Work out the finished part from the listing and answer in its coordinate system (mm). Give positions to 0.01 mm unless a question says otherwise; leave off trailing zeros. Write each loop counter-clockwise with the first axis right and the second up, starting at its lowest first coordinate (ties: lowest second). Pieces come first, ordered by that corner, then holes. Notation, with made-up numbers: (38, 85) -> (46, 85) arc R21 ccw to (46, 118) -> close; hole circle Ø2 at (-8.75, 43.25). An arc over 180 degrees is marked (long way). Use a Markdown table: item, result. Add a question column.
Q1. For a pull along Y with two mould halves and no side action, classify faces 1 (the face through (-11.012, -49.592, 3.131)), 2 (the face through (-1, 1, 0)), 3 (the face through (36, -8.466, 3)), 4 (the face through (12, -29.209, 3)) as pulls with the +Y half, pulls with the -Y half, needs draft (parallel to the pull), parting line crosses it, or undercut.
Q2. Section A-A, the plane x = 0 is taken. Give the vertices of the cut face in (y, z), plus the area to 3 significant figures.
Q3. Section C-C, the plane y = 17 is taken. Give the vertices of the cut face in (x, z), plus the area to 3 significant figures.
Q4. Consider line 1 (Y direction, x = 15.5, z = 1); line 2 (Y direction, x = 29.5, z = 3.25); line 3 (Y direction, x = 38, z = 3.75). Determine where each line is inside the solid, lowest interval first.
Q5. Each of these flat-tipped pins is pushed along its axis until it touches: pin 1 Ø3 at (x, z) = (35, 3.5) entering from +Y; pin 2 Ø3 at (y, z) = (19.5, 4) entering from -X; pin 3 Ø2 at (x, z) = (-18.5, 4.5) entering from +Y. Where does it stop, or does it pass through?
Q6. Section D-D, the plane x = 11 is taken. Give the vertices of the cut face in (y, z), plus the area to 3 significant figures.
Q7. Section B-B, the plane z = 4.25 is taken. State how many separate pieces and enclosed holes the cut face has, plus the area to 3 significant figures.
from build123d import *

# Parameters (mm, degrees)
SKETCH1_R           = 50.8
BOSS_EXTRUDE1_DEPTH = 6.35
SKETCH2_W           = 19.230854478
SKETCH2_H           = 28.543909792
SKETCH2_W_2         = 18.081841161
SKETCH2_H_2         = 27.999640326
SKETCH2_W_3         = 10.22017109
SKETCH2_H_3         = 7.559298144
SKETCH2_W_4         = 8.829260232
SKETCH2_H_4         = 7.256926218
SKETCH2_W_5         = 9.97827355
SKETCH2_H_5         = 8.164041996
SKETCH2_W_6         = 10.703966172
SKETCH2_H_6         = 6.531233596
SKETCH2_W_7         = 12.336774571
SKETCH2_H_7         = 9.04092058
SKETCH2_W_8         = 11.127286868
SKETCH2_H_8         = 7.7407213
CUT_EXTRUDE1_DEPTH  = 73.122135992


with BuildPart() as part:
    # Sketch1 → Boss-Extrude1 (new body)
    with BuildSketch(Plane.XY):
        Circle(SKETCH1_R)
    extrude(amount=BOSS_EXTRUDE1_DEPTH)

    # Sketch2 → Cut-Extrude1 (cut, through all)
    with BuildSketch(Plane.XY.offset(6.35)):
        with Locations((-19.896072715, 17.295674154)):
            Rectangle(SKETCH2_W, SKETCH2_H)
        with Locations((23.736196173, 16.963065035)):
            Rectangle(SKETCH2_W_2, SKETCH2_H_2)
        with Locations((-29.541737147, -18.77729659)):
            Rectangle(SKETCH2_W_3, SKETCH2_H_3)
        with Locations((-18.505161857, -29.209128029)):
            Rectangle(SKETCH2_W_4, SKETCH2_H_4)
        with Locations((-3.235379606, -36.919612136)):
            Rectangle(SKETCH2_W_5, SKETCH2_H_5)
        with Locations((12.548434919, -32.474744827)):
            Rectangle(SKETCH2_W_6, SKETCH2_H_6)
        with Locations((25.822562461, -23.29775688)):
            Rectangle(SKETCH2_W_7, SKETCH2_H_7)
        with Locations((35.740361625, -12.336774571)):
            Rectangle(SKETCH2_W_8, SKETCH2_H_8)
    extrude(amount=-CUT_EXTRUDE1_DEPTH, mode=Mode.SUBTRACT)


solid = part.part
Result set:
| question | item | result |
|---|---|---|
| 1 | face 1 | parting line crosses it |
| 1 | face 2 | needs draft |
| 1 | face 3 | undercut |
| 1 | face 4 | undercut |
| 2 | outline | (-50.8, 0) -> (-41, 0) -> (-41, 6.35) -> (-50.8, 6.35) -> close; (-32.84, 0) -> (50.8, 0) -> (50.8, 6.35) -> (-32.84, 6.35) -> close |
| 2 | area | 593 mm2 |
| 3 | outline | (-47.87, 0) -> (-29.51, 0) -> (-29.51, 6.35) -> (-47.87, 6.35) -> close; (-10.28, 0) -> (14.7, 0) -> (14.7, 6.35) -> (-10.28, 6.35) -> close; (32.78, 0) -> (47.87, 0) -> (47.87, 6.35) -> (32.78, 6.35) -> close |
| 3 | area | 371 mm2 |
| 4 | line 1 | y = -48.38 to -35.74, -29.21 to 2.96, 30.96 to 48.38 |
| 4 | line 2 | y = -41.36 to -27.82, -18.78 to 2.96, 30.96 to 41.36 |
| 4 | line 3 | y = -33.71 to -16.21, -8.47 to 33.71 |
| 5 | pin 1 | stops at y = 38.19 |
| 5 | pin 2 | stops at x = -47.5 |
| 5 | pin 3 | stops at y = 47.69 |
| 6 | outline | (-49.59, 0) -> (-35.74, 0) -> (-35.74, 6.35) -> (-49.59, 6.35) -> close; (-29.21, 0) -> (49.59, 0) -> (49.59, 6.35) -> (-29.21, 6.35) -> close |
| 6 | area | 588 mm2 |
| 7 | separate pieces | 1 |
| 7 | enclosed holes | 8 |
| 7 | area | 6,560 mm2 |
